Source: three-view drawing plus pictorial views. Frame: mm from the lowest corner of the part. Give positions to 0.01 mm unless a question says otherwise; leave off trailing zeros. Loops run counter-clockwise (first coordinate to the right, second up) from the corner with the lowest first, then second, coordinate; pieces in that order, holes last. Notation, with made-up numbers: M -9.5,16.25 L -0.5,16.25 A11 cw -0.5,20.25 Z; hole C 23,-16 d11. An arc over 180 degrees is marked long. One line per item, written item: value. Start each with the question number.
(1) Section D-D on x = 24. Output: boundary loops of the cut face in (y, z).
(2) Section C-C on y = 21. Output: boundary loops of the cut face in (x, z), plus the area to 3 significant figures.
(3) Section A-A on z = 8.75. Output: boundary loops of the cut face in (x, y), plus the area to 3 significant figures.
(4) Section B-B on x = 70.75. Output: boundary loops of the cut face in (y, z).
(5) Pull-direction query (Z, two-part tool) for the marked faces 1, 2 and 3; classes: released by +Z, released by -Z, zero draft, split by the parting line, or undercut.
(6) Pin query (flat end, axial travel): P1, Ø2, axis at y = 12, z = 15, coming from the -X side; P2, Ø1.8, axis at x = 40, y = 21, coming from the +Z side. Return the tip coordinate at first contact, or that it passes through.
(7) Ray query, line 1 along X through (y, z) = (21, 18.5); line 2 along Y through (x, z) = (56, 10); line 3 along X through (y, z) = (28.5, 6.5). Return the intervals inside material, ascending. Write a range as from..to.
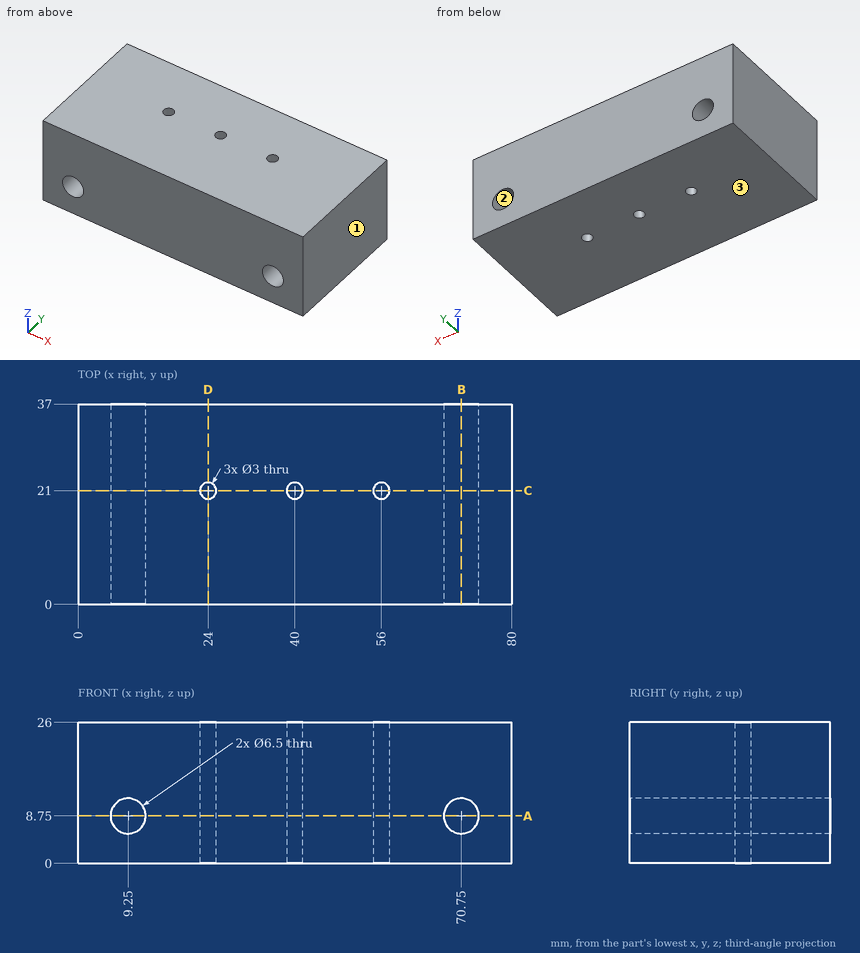
Output values:
1. outline: M 0,0 L 19.5,0 L 19.5,26 L 0,26 Z; M 22.5,0 L 37,0 L 37,26 L 22.5,26 Z
2. outline: M 0,0 L 22.5,0 L 22.5,26 L 0,26 Z; M 25.5,0 L 38.5,0 L 38.5,26 L 25.5,26 Z; M 41.5,0 L 54.5,0 L 54.5,26 L 41.5,26 Z; M 57.5,0 L 80,0 L 80,26 L 57.5,26 Z; hole C 9.25,8.75 d6.5; hole C 70.75,8.75 d6.5
2. area: 1,780 mm²
3. outline: M 0,0 L 6,0 L 6,37 L 0,37 Z; M 12.5,0 L 67.5,0 L 67.5,37 L 12.5,37 Z; M 74,0 L 80,0 L 80,37 L 74,37 Z; hole C 24,21 d3; hole C 40,21 d3; hole C 56,21 d3
3. area: 2,460 mm²
4. outline: M 0,0 L 37,0 L 37,5.5 L 0,5.5 Z; M 0,12 L 37,12 L 37,26 L 0,26 Z
5. face 1: zero draft
5. face 2: undercut
5. face 3: released by -Z
6. P1: stops at x = 0
6. P2: passes through
7. line 1: x = 0..22.5, 25.5..38.5, 41.5..54.5, 57.5..80
7. line 2: y = 0..19.5, 22.5..37
7. line 3: x = 0..6.9, 11.6..68.4, 73.1..80
